Input: part model. Units: mm. Frame: model coordinates. A direction names the side the tool comes from. Coordinates: 2 decimals unless noted, no trailing zeros. Write each loop counter-clockwise with the first axis right and the second up, starting at its lowest first coordinate (ties: lowest second). Pieces come first, ordered by that corner, then holes. Notation, with made-up numbers: M -23.75,67.25 L 25.25,67.25 A26 ccw 25.25,100.25 Z; hole C 1.25,59 d7. An arc over 180 degrees is marked long. Use one line per item in the form item = value.
from build123d import *

# Parameters (mm, degrees)
CYLINDER006_R        = 1.9
CYLINDER006_DEPTH    = 10
ARRAY_X_COUNT        = 2
ARRAY_X_PITCH        = 31
ARRAY_Y_COUNT        = 2
ARRAY_Y_PITCH        = 31
CYLINDER009_R        = 2.1
CYLINDER009_DEPTH    = 10
ARRAY002_X_COUNT     = 3
ARRAY002_X_PITCH     = 10
ARRAY002_Y_COUNT     = 2
ARRAY002_Y_PITCH     = 10
BODY_PITCH_ANGLE     = -90
BODY_PLACEMENT_ANGLE = -90
CYLINDER005_R        = 14
CYLINDER005_DEPTH    = 20
PAD_DEPTH            = 5
BOX004_W             = 24
BOX004_H             = 7
BOX004_DEPTH         = 30
FILLET004_R          = 3
BOX003_W             = 54
BOX003_H             = 46
BOX003_DEPTH         = 5
FILLET001_R          = 5


with BuildPart() as stepper_bolt_hole_array:
    # Cylinder006 → Cylinder006 (new body)
    with BuildSketch(Plane(origin=(0, 38, 0), x_dir=(1, 0, 0), z_dir=(0, 0, 1))):
        Circle(CYLINDER006_R)
    extrude(amount=CYLINDER006_DEPTH)

    # Array X: stepper bolt hole array ×2


with BuildPart() as stepper_bolt_hole_array_1:
    add(stepper_bolt_hole_array.part)
    with Locations(*[(i * ARRAY_X_PITCH, 0, 0) for i in range(1, ARRAY_X_COUNT)]):
        add(stepper_bolt_hole_array.part)

    # Array Y: stepper bolt hole array ×2


with BuildPart() as stepper_bolt_hole_array_2:
    add(stepper_bolt_hole_array_1.part)
    with Locations(*[(0, i * ARRAY_Y_PITCH, 0) for i in range(1, ARRAY_Y_COUNT)]):
        add(stepper_bolt_hole_array_1.part)


with BuildPart() as stepper_bolt_hole_array_3:
    # Array placement: moved
    add(stepper_bolt_hole_array_2.part.moved(Location((-15.5, -15.5, 0))))


with BuildPart() as obj1:
    # Cylinder009 → Cylinder009 (new body)
    with BuildSketch(Plane.XY):
        Circle(CYLINDER009_R)
    extrude(amount=CYLINDER009_DEPTH)

    # Array002 X: obj1_3


with BuildPart() as obj1_1:
    add(obj1.part)
    with Locations(*[(i * ARRAY002_X_PITCH, 0, 0) for i in range(1, ARRAY002_X_COUNT)]):
        add(obj1.part)

    # Array002 Y: obj1_2


with BuildPart() as obj1_2:
    add(obj1_1.part)
    with Locations(*[(0, i * ARRAY002_Y_PITCH, 0) for i in range(1, ARRAY002_Y_COUNT)]):
        add(obj1_1.part)


with BuildPart() as obj1_3:
    # Body pitch: moved
    add(obj1_2.part.rotate(Axis((0, 0, 0), (0, 1, 0)), BODY_PITCH_ANGLE))


with BuildPart() as obj1_4:
    # Body placement: moved
    add(obj1_3.part.moved(Location((-45, 0, 5))).rotate(Axis((-45, 0, 5), (0, 0, 1)), BODY_PLACEMENT_ANGLE))


with BuildPart() as part_mirroring005:
    # Part__Mirroring005: instance of obj1
    add(obj1_4.part.mirror(Plane(origin=(0, 0, 0), x_dir=(0, -1, 0), z_dir=(1, 0, 0))))


with BuildPart() as stepper_wall_extract_fusion:
    # Cylinder005 → Cylinder005 (new body)
    with BuildSketch(Plane(origin=(0, 38, 0), x_dir=(1, 0, 0), z_dir=(0, 0, 1))):
        Circle(CYLINDER005_R)
    extrude(amount=CYLINDER005_DEPTH)

    # Fusion006: union stepper bolt hole array, Part__Mirroring005, obj1
    add(stepper_bolt_hole_array_3.part)
    add(part_mirroring005.part)
    add(obj1_4.part)


with BuildPart() as side_body:
    # Sketch → Pad (new body)
    with BuildSketch(Plane.YZ):
        Polygon((50, 0), (0, 0), (0, 30), (7, 30), align=None)
    extrude(amount=-PAD_DEPTH)


with BuildPart() as side_body_1:
    # Body001 placement: moved
    add(side_body.part.moved(Location((27, 0, 0))))


with BuildPart() as side_body_fusion:
    # Part__Mirroring002: instance of side body
    add(side_body_1.part.mirror(Plane(origin=(0, 0, 0), x_dir=(0, -1, 0), z_dir=(1, 0, 0))))

    # Fusion009: union side body
    add(side_body_1.part)


with BuildPart() as stepper_top_wall_fillet:
    # Box004 → Box004 (new body)
    with BuildSketch(Plane(origin=(27, 0, 0), x_dir=(1, 0, 0), z_dir=(0, 0, 1))):
        with Locations((12, 3.5)):
            Rectangle(BOX004_W, BOX004_H)
    extrude(amount=BOX004_DEPTH)

    # Fillet004
    fillet004_edges = [stepper_top_wall_fillet.edges().sort_by_distance(p)[0] for p in [
        (51, 3.5, 30),
        (51, 3.5, 0),
    ]]
    fillet(fillet004_edges, radius=FILLET004_R)


with BuildPart() as part_mirroring003:
    # Part__Mirroring003: instance of stepper top wall fillet
    add(stepper_top_wall_fillet.part.mirror(Plane(origin=(0, 0, 0), x_dir=(0, -1, 0), z_dir=(1, 0, 0))))


with BuildPart() as stepper_holder_cut:
    # Box003 → Box003 (new body)
    with BuildSketch(Plane(origin=(-27, 15, 0), x_dir=(1, 0, 0), z_dir=(0, 0, 1))):
        with Locations((27, 23)):
            Rectangle(BOX003_W, BOX003_H)
    extrude(amount=BOX003_DEPTH)

    # Fillet001
    fillet001_edges = [stepper_holder_cut.edges().sort_by_distance(p)[0] for p in [
        (-27, 61, 2.5),
        (27, 61, 2.5),
    ]]
    fillet(fillet001_edges, radius=FILLET001_R)

    # Fusion007: union stepper top wall fillet, Part__Mirroring003
    add(stepper_top_wall_fillet.part)
    add(part_mirroring003.part)

    # Fusion010: union side body fusion
    add(side_body_fusion.part)

    # Cut004002: cut stepper wall extract fusion
    add(stepper_wall_extract_fusion.part, mode=Mode.SUBTRACT)


solid = stepper_holder_cut.part
(1) First-contact query: pin 1 Ø4 at (x, z) = (3.5, 3.5) entering from -Y; pin 2 Ø14 at (x, y) = (11, 33.5) entering from +Z; pin 3 Ø12 at (y, z) = (10, 4.5) entering from +X; pin 4 Ø5 at (x, z) = (45, 5) entering from +Y. Flat tips, straight axial feed; report the tip coordinate or a pass-through.
Computed:
pin_1 = 15
pin_2 = 5
pin_3 = 51
pin_4 = 7
(2) Pull-direction query (X, two-part tool) for faces 3 (the cylindrical face through (47.05, 3.45, 14.54)), 4 (the flat face through (-39, 7, 15)), 5 (the flat face through (51, 3, 15)); classes: pulls with the +X half, pulls with the -X half, needs draft (parallel to the pull), parting line crosses it, or undercut.
Computed:
face_3 = undercut
face_4 = needs draft
face_5 = pulls with the +X half
(3) Set-up query: faces 1 (the cylindrical face through (50.14, 3.55, 29.1)), 2 (the flat face through (27, 26, 8)). Return all of +Z, -Z, +X, -X, +Y, -Y with unobstructed straight access to the full face (end or side cutting, diameter ignored); none if empty.
Computed:
face_1 = +Z, +X, +Y, -Y
face_2 = +Z, -Z, +X, +Y
(4) Section query D-D on y = 53.5. Return the cut outline in (x, z).
Computed:
outline = M -27,0 L -17.4,0 L -17.4,5 L -27,5 Z; M -13.6,0 L 13.6,0 L 13.6,5 L -13.6,5 Z; M 17.4,0 L 27,0 L 27,5 L 17.4,5 Z
(5) Line query: probe 1 along Z at (x, y) = (-35, 5.5); probe 2 along X at (y, z) = (3.5, 15); probe 3 along Y at (x, z) = (15.5, 3.45). Output: solid intervals per line, ascending.
Computed:
probe_1 = 0 to 2.9, 7.1 to 12.9, 17.1 to 22.9, 27.1 to 30
probe_2 = -51 to -47.1, -42.9 to -37.1, -32.9 to -22, 22 to 32.9, 37.1 to 42.9, 47.1 to 51
probe_3 = 15 to 20.6, 24.4 to 51.6, 55.4 to 61
(6) Section query C-C on z = 9. Return the cut outline in (x, y), plus the area to 3 significant figures.
Computed:
outline = M -51,0 L -22,0 L -22,37.1 L -27,37.1 L -27,7 L -51,7 Z; M 22,0 L 51,0 L 51,7 L 27,7 L 27,37.1 L 22,37.1 Z
area = 707 mm^2
(7) Section query A-A on z = 15. Return the cut outline in (x, y).
Computed:
outline = M -51,0 L -47.1,0 L -47.1,7 L -51,7 Z; M -42.9,0 L -37.1,0 L -37.1,7 L -42.9,7 Z; M -32.9,0 L -22,0 L -22,28.5 L -27,28.5 L -27,7 L -32.9,7 Z; M 22,0 L 32.9,0 L 32.9,7 L 27,7 L 27,28.5 L 22,28.5 Z; M 37.1,0 L 42.9,0 L 42.9,7 L 37.1,7 Z; M 47.1,0 L 51,0 L 51,7 L 47.1,7 Z
(8) Section query B-B on x = 15.5. Return the cut outline in (y, z), plus the area to 3 significant figures.
Computed:
outline = M 15,0 L 20.6,0 L 20.6,5 L 15,5 Z; M 24.4,0 L 51.6,0 L 51.6,5 L 24.4,5 Z; M 55.4,0 L 61,0 L 61,5 L 55.4,5 Z
area = 192 mm^2
